For this review, take the finished solid that the model builds, in its own axes (mm). Face numbers are marked on the shaded views. A direction names the side the tool comes from. Give positions to 0.01 mm unless a question says otherwise; leave off trailing zeros. Loops run counter-clockwise (first coordinate to the right, second up) from the corner with the lowest first, then second, coordinate; pieces in that order, holes last.
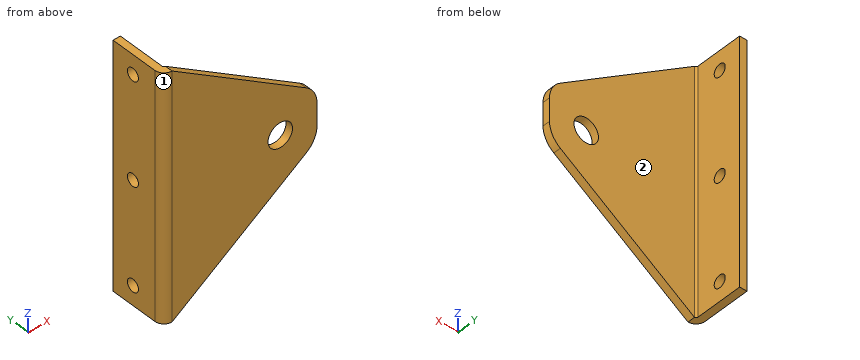
```python
from build123d import *

# Parameters (mm, degrees)
BASE_FLANGE1_DEPTH = 100
CUT_EXTRUDE1_REACH = 120.322
SKETCH6_R          = 2.55
CUT_EXTRUDE2_REACH = 120.322
SKETCH7_R          = 5
CUT_EXTRUDE4_DEPTH = 10


# Sheet-metal steps are written as plain solids
with BuildPart() as part:
    # Sketch1 → Base-Flange1 (new body)
    with BuildSketch(Plane.XY):
        with BuildLine():
            Line((0, 20), (0, 0.7366))
            ThreePointArc((0, 0.7366), (0.215745145, 0.215745145), (0.7366, 0))
            Line((0.7366, 0), (60, 0))
            Line((60, 0), (60, -3))
            Line((60, -3), (0.7366, -3))
            ThreePointArc((0.7366, -3), (-1.905575199, -1.905575199), (-3, 0.7366))
            Line((-3, 0.7366), (-3, 20))
            Line((-3, 20), (0, 20))
        make_face()
    extrude(amount=BASE_FLANGE1_DEPTH)

    # Sketch6 → Cut-Extrude1 (cut, up to next)
    with BuildSketch(Plane(origin=(0, 0, 0), x_dir=(0, 0, -1), z_dir=(1, 0, 0)), mode=Mode.PRIVATE) as cut_extrude1_sk1:
        with Locations(Location((-92, 10.813082186, 0), (0, 0, 90))):
            Circle(SKETCH6_R)
    cut_extrude1_tool1 = extrude(cut_extrude1_sk1.sketch, amount=-CUT_EXTRUDE1_REACH, mode=Mode.PRIVATE) & part.part
    # Sketch6 → Cut-Extrude1 (cut, up to next)
    with BuildSketch(Plane(origin=(0, 0, 0), x_dir=(0, 0, -1), z_dir=(1, 0, 0)), mode=Mode.PRIVATE) as cut_extrude1_sk2:
        with Locations(Location((-8, 10.813082186, 0), (0, 0, 90))):
            Circle(SKETCH6_R)
    cut_extrude1_tool2 = extrude(cut_extrude1_sk2.sketch, amount=-CUT_EXTRUDE1_REACH, mode=Mode.PRIVATE) & part.part
    # Sketch6 → Cut-Extrude1 (cut, up to next)
    with BuildSketch(Plane(origin=(0, 0, 0), x_dir=(0, 0, -1), z_dir=(1, 0, 0)), mode=Mode.PRIVATE) as cut_extrude1_sk3:
        with Locations(Location((-50, 10.813082186, 0), (0, 0, 90))):
            Circle(SKETCH6_R)
    cut_extrude1_tool3 = extrude(cut_extrude1_sk3.sketch, amount=-CUT_EXTRUDE1_REACH, mode=Mode.PRIVATE) & part.part
    add(cut_extrude1_tool1.solids().sort_by_distance((0, 10.813082, 92))[0], mode=Mode.SUBTRACT)
    add(cut_extrude1_tool2.solids().sort_by_distance((0, 10.813082, 8))[0], mode=Mode.SUBTRACT)
    add(cut_extrude1_tool3.solids().sort_by_distance((0, 10.813082, 50))[0], mode=Mode.SUBTRACT)

    # Sketch7 → Cut-Extrude2 (cut, up to next)
    with BuildSketch(Plane(origin=(0, 0, 0), x_dir=(1, 0, 0), z_dir=(0, 1, 0)), mode=Mode.PRIVATE) as cut_extrude2_sk1:
        with Locations(Location((45, -50, 0), (0, 0, 270))):
            Circle(SKETCH7_R)
    cut_extrude2_tool1 = extrude(cut_extrude2_sk1.sketch, amount=-CUT_EXTRUDE2_REACH, mode=Mode.PRIVATE) & part.part
    add(cut_extrude2_tool1.solids().sort_by_distance((45, 0, 50))[0], mode=Mode.SUBTRACT)

    # Sketch8 → Cut-Extrude4 (cut)
    with BuildSketch(Plane(origin=(0, 0, 0), x_dir=(1, 0, 0), z_dir=(0, 1, 0))):
        with BuildLine():
            Line((0.7366, 0), (55.594459994, -37.026468271))
            ThreePointArc((55.594459994, -37.026468271), (58.830192522, -40.621768617), (60, -45.315136281))
            Line((60, -45.315136281), (60, -54.684863719))
            ThreePointArc((60, -54.684863719), (58.830192522, -59.378231383), (55.594459994, -62.973531729))
            Line((55.594459994, -62.973531729), (0.7366, -100))
            Line((0.7366, -100), (64.682636993, -100))
            Line((64.682636993, -100), (64.682636993, 0))
            Line((64.682636993, 0), (0.7366, 0))
        make_face()
    extrude(amount=-CUT_EXTRUDE4_DEPTH, mode=Mode.SUBTRACT)


solid = part.part
```
Item 1: Take a section at A-A on z = 50. Give the boundary of the cut face in (x, y).
Answer:
outline: (-3, 0.74) arc R3.74 ccw to (0.74, -3) - (40, -3) - (40, 0) - (0.74, 0) arc R0.74 cw to (0, 0.74) - (0, 8.26) - (-3, 8.26) - close; (-3, 13.36) - (0, 13.36) - (0, 20) - (-3, 20) - close; (50, -3) - (60, -3) - (60, 0) - (50, 0) - close
Item 2: For L1, parallel to X at y = 11.25, z = 80; L2, parallel to X at y = -1.8, z = 50, list the stretches that pass through material, from the lowest coordinate up.
Answer:
L1: x = -3 to 0
L2: x = -2.01 to 40, 50 to 60
Item 3: Take a section at B-B on z = 8. Give the boundary of the cut face in (x, y).
Answer:
outline: (-3, 0.74) arc R3.74 ccw to (0.74, -3) - (12.59, -3) - (12.59, 0) - (0.74, 0) arc R0.74 cw to (0, 0.74) - (0, 8.26) - (-3, 8.26) - close; (-3, 13.36) - (0, 13.36) - (0, 20) - (-3, 20) - close
Item 4: Take a section at C-C on x = 45. Give the boundary of the cut face in (y, z), and give its area (3 significant figures).
Answer:
outline: (-3, 29.88) - (0, 29.88) - (0, 45) - (-3, 45) - close; (-3, 55) - (0, 55) - (0, 70.12) - (-3, 70.12) - close
area: 90.7 mm2
Item 5: Take a section at D-D on y = 2. Give the boundary of the cut face in (x, z), and give its area (3 significant figures).
Answer:
outline: (-3, 0) - (0, 0) - (0, 100) - (-3, 100) - close
area: 300 mm2
Item 6: Clearance check with flat-ended pins moving along their axes: pin 1 Ø10 at (x, z) = (16, 59) entering from +Y; pin 2 Ø2 at (y, z) = (7.5, 64.5) entering from +X. State where each tip first meets the part, or that it passes through.
Answer:
pin 1: stops at y = 0
pin 2: stops at x = 0
Item 7: Tool access review of the marked faces 1 and 2: name each direction out of +Z, -Z, +X, -X, +Y, -Y from which nothing blocks a thin tool from reaching the whole face with its end or side.
Answer:
face 1: +Z, -Z, -X, -Y
face 2: +Z, -Z, +X, +Y
